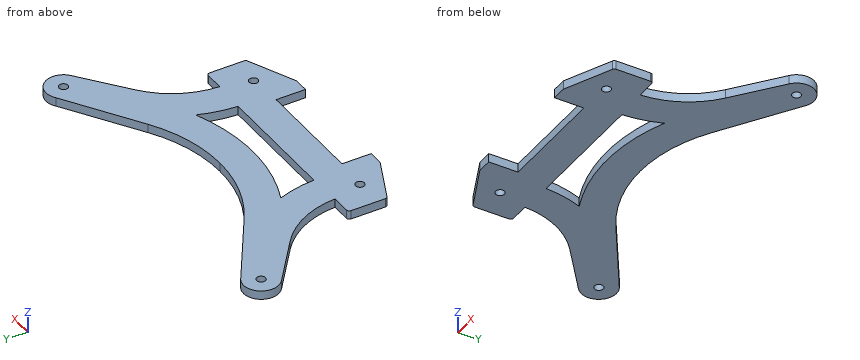
Autodesk Inventor part; units mm, degrees
ref_plane "Plano de trabajo1" through (20.4772, 21.1232, 0) normal (-1, 0, 0) x (0, 0, 1)
ref_plane "YZ Plane" through (0, 0, 0) normal (1, 0, 0) x (0, 1, 0)
ref_plane "XZ Plane" through (0, 0, 0) normal (0, 1, 0) x (-1, 0, 0)
sketch "Boceto1" plane through (0, 0, 0) normal (0, 0, 1) x (1, 0, 0)
  line L0 (20.4772, 24.8969) -> (57.9772, 24.8969)
  line L1 (86.0741, 43.5717) -> (86.0741, 43.5717)
  arc A0 (108.9954, 90.7434) -> (86.144, 46.4672) centre (146.0741, 43.5717) ccw
  arc A1 (20.4772, 85.7499) -> (75.1704, 101.8402) centre (20.4772, 186.7499) ccw
  line L2 (108.9954, 90.7434) -> (140.4433, 115.4625)
  arc A2 (140.4433, 115.4625) -> (125.6118, 134.3312) centre (133.0275, 124.8969) ccw
  line L3 (125.6118, 134.3312) -> (75.1704, 101.8402)
  line L4 (57.9772, 24.8969) -> (57.9772, 4.8969)
  line L5 (57.9772, 4.8969) -> (67.9772, 4.8969)
  line L6 (67.9772, 4.8969) -> (99.8761, 19.3004)
  line L7 (101.053, 21.1232) -> (101.053, 44.4672)
  line L8 (99.053, 46.4672) -> (86.144, 46.4672)
  line L9 (20.4772, -46.5022) -> (20.4772, 138.2428)
  arc A3 (101.053, 44.4672) -> (99.053, 46.4672) centre (99.053, 44.4672) ccw
  arc A4 (99.8761, 19.3004) -> (101.053, 21.1232) centre (99.053, 21.1232) ccw
  line L10 (20.4772, 24.8969) -> (-17.0228, 24.8969)
  line L11 (-45.1197, 43.5717) -> (-45.1197, 43.5717)
  arc A5 (-45.1896, 46.4672) -> (-68.041, 90.7434) centre (-105.1197, 43.5717) ccw
  arc A6 (-34.216, 101.8402) -> (20.4772, 85.7499) centre (20.4772, 186.7499) ccw
  line L12 (-68.041, 90.7434) -> (-99.4888, 115.4625)
  arc A7 (-84.6574, 134.3312) -> (-99.4888, 115.4625) centre (-92.0731, 124.8969) ccw
  line L13 (-84.6574, 134.3312) -> (-34.216, 101.8402)
  line L14 (-17.0228, 24.8969) -> (-17.0228, 4.8969)
  line L15 (-17.0228, 4.8969) -> (-27.0228, 4.8969)
  line L16 (-27.0228, 4.8969) -> (-58.9217, 19.3004)
  line L17 (-60.0986, 21.1232) -> (-60.0986, 44.4672)
  line L18 (-58.0986, 46.4672) -> (-45.1896, 46.4672)
  arc A8 (-58.0986, 46.4672) -> (-60.0986, 44.4672) centre (-58.0986, 44.4672) ccw
  arc A9 (-60.0986, 21.1232) -> (-58.9217, 19.3004) centre (-58.0986, 21.1232) ccw
  point P0 (0, 0)
  dimension "d0" = 37.5
  dimension "d1" = 60
  dimension "d3" = 40
  dimension "d4" = 12
  dimension "d5" = 60
  dimension "d6" = 101
  dimension "d7" = 2
  dimension "d21" = 10
  dimension "d23" = 35
  dimension "d42" = 100
  dimension "d43" = 20
extrude "Extrusión1" add sketch "Boceto1" along normal blind 6
hole "Agujero1" at (-40.0986, 26.4672, 6) direction (0, 0, -1) diameter 6 end through all
ref_plane "Plano de trabajo1" through (20.4772, 21.1232, 0) normal (-1, 0, 0) x (0, 0, 1)
mirror "Simetría1" about plane through (20.4772, 21.1232, 0) normal (-1, 0, 0) of "Agujero1"
hole "Agujero2" at (-92.0731, 124.8969, 6) direction (0, 0, -1) diameter 6 end through all
hole "Agujero3" at (133.0275, 124.8969, 6) direction (0, 0, -1) diameter 6 end through all
sketch "Boceto3" plane through (0, 0, 6) normal (0, 0, 1) x (1, 0, 0)
  circle A0 centre (133.0275, 124.8969) radius 3
  circle A1 centre (-92.0731, 124.8969) radius 3
  circle A2 centre (81.053, 26.4672) radius 3
  circle A3 centre (-40.0986, 26.4672) radius 3
  arc A4 (-34.216, 101.8402) -> (75.1704, 101.8402) centre (20.4772, 186.7499) ccw
  line L0 (-34.216, 101.8402) -> (-84.6574, 134.3312)
  arc A5 (-84.6574, 134.3312) -> (-99.4888, 115.4625) centre (-92.0731, 124.8969) ccw
  line L1 (-99.4888, 115.4625) -> (-68.041, 90.7434)
  arc A6 (-45.1896, 46.4672) -> (-68.041, 90.7434) centre (-105.1197, 43.5717) ccw
  line L2 (-45.1896, 46.4672) -> (-58.0986, 46.4672)
  arc A7 (-58.0986, 46.4672) -> (-60.0986, 44.4672) centre (-58.0986, 44.4672) ccw
  line L3 (-60.0986, 44.4672) -> (-60.0986, 21.1232)
  arc A8 (-60.0986, 21.1232) -> (-58.9217, 19.3004) centre (-58.0986, 21.1232) ccw
  line L4 (-58.9217, 19.3004) -> (-27.0228, 4.8969)
  line L5 (-27.0228, 4.8969) -> (-17.0228, 4.8969)
  line L6 (-17.0228, 4.8969) -> (-17.0228, 24.8969)
  line L7 (-17.0228, 24.8969) -> (57.9772, 24.8969)
  line L8 (57.9772, 24.8969) -> (57.9772, 4.8969)
  line L9 (57.9772, 4.8969) -> (67.9772, 4.8969)
  line L10 (67.9772, 4.8969) -> (99.8761, 19.3004)
  arc A9 (99.8761, 19.3004) -> (101.053, 21.1232) centre (99.053, 21.1232) ccw
  line L11 (101.053, 21.1232) -> (101.053, 44.4672)
  arc A10 (101.053, 44.4672) -> (99.053, 46.4672) centre (99.053, 44.4672) ccw
  line L12 (99.053, 46.4672) -> (86.144, 46.4672)
  arc A11 (108.9954, 90.7434) -> (86.144, 46.4672) centre (146.0741, 43.5717) ccw
  line L13 (108.9954, 90.7434) -> (140.4433, 115.4625)
  arc A12 (140.4433, 115.4625) -> (125.6118, 134.3312) centre (133.0275, 124.8969) ccw
  line L14 (125.6118, 134.3312) -> (75.1704, 101.8402)
  arc A13 (-28.0705, 73.1557) -> (69.0249, 73.1557) centre (20.4772, 186.7499) ccw
  arc A14 (-22.6764, 47.4304) -> (-28.0705, 73.1557) centre (-105.1197, 43.5717) ccw
  line L15 (-22.6764, 47.4304) -> (63.6308, 47.4304)
  arc A15 (69.0249, 73.1557) -> (63.6308, 47.4304) centre (146.0741, 43.5717) ccw
  point P0 (0, 0)
extrude "Extrusión3" cut sketch "Boceto3" against normal through all contours A13 A15 L15 A14
properties part number "back_plate"
Build history of the part. All positions in model axes, mm. Give positions to 0.01 mm unless a question says otherwise; leave off trailing zeros. Loops run counter-clockwise (first coordinate to the right, second up) from the corner with the lowest first, then second, coordinate; pieces in that order, holes last. Notation, with made-up numbers: (10, -19) - (34, -19) arc R27 ccw to (34, 10) - close; hole circle Ø10 at (81, -14). An arc over 180 degrees is marked (long way). Use a Markdown table: item, result.
(1) Band-saw the part on B-B (y = 52.5). Give the cut face in (x, z).
Taken from the geometry:
| item | result |
|---|---|
| outline | (-45.79, 0) - (-23.07, 0) - (-23.07, 6) - (-45.79, 6) - close; (64.02, 0) - (86.74, 0) - (86.74, 6) - (64.02, 6) - close |
(2) Drop flat-ended pins along their axis: pin 1 Ø12 at (x, y) = (56, 72) entering from -Z; pin 2 Ø3 at (x, z) = (40, 2) entering from +Y; pin 3 Ø1 at (x, z) = (-13, 2.5) entering from +Y; pin 4 Ø1 at (y, z) = (37, 1.5) entering from -X. Give the stop position or say it passes through.
Taken from the geometry:
| item | result |
|---|---|
| pin 1 | z = 0 |
| pin 2 | y = 87.96 |
| pin 3 | y = 91.64 |
| pin 4 | x = -60.1 |
(3) Wall check: line 1 along X through (y, z) = (26, 4); line 2 along X through (y, z) = (56.5, 3.2) (1 decimal); line 3 along X through (y, z) = (117.5, 4.05). Give the ranges that are in metal, low to high.
Taken from the geometry:
| item | result |
|---|---|
| line 1 | -60.1 to -43.06, -37.14 to 78.09, 84.02 to 101.05 |
| line 2 | -46.5 to -23.6, 64.6 to 87.5 |
| line 3 | -101.52 to -58.53, 99.48 to 142.48 |
(4) Band-saw the part on D-D (y = 125). Give the cut face in (x, z), and give its area (3 significant figures).
Taken from the geometry:
| item | result |
|---|---|
| outline | (-104.07, 0) - (-95.07, 0) - (-95.07, 6) - (-104.07, 6) - close; (-89.07, 0) - (-70.17, 0) - (-70.17, 6) - (-89.07, 6) - close; (111.13, 0) - (130.03, 0) - (130.03, 6) - (111.13, 6) - close; (136.03, 0) - (145.03, 0) - (145.03, 6) - (136.03, 6) - close |
| area | 335 mm2 |
(5) Band-saw the part on A-A (x = 32). Give the cut face in (y, z) (3 decimals).
Taken from the geometry:
| item | result |
|---|---|
| outline | (24.897, 0) - (47.43, 0) - (47.43, 6) - (24.897, 6) - close; (63.755, 0) - (86.409, 0) - (86.409, 6) - (63.755, 6) - close |
(6) Band-saw the part on C-C (z = 4.1). Give the number of separate pieces and of enclosed holes in the cut face, and give its area (3 significant figures).
Taken from the geometry:
| item | result |
|---|---|
| separate pieces | 1 |
| enclosed holes | 5 |
| area | 12,800 mm2 |
